Part model, mm, in its own coordinate system. Coordinates: 2 decimals unless noted, no trailing zeros. Order: outer loops, then holes, each group sorted by start corner. A loop starts at its lowest first (then second) coordinate and runs counter-clockwise, first axis right, second up.
1) Pin check, flat tips, straight feed: pin 1 Ø1 at (y, z) = (0, 2.5) entering from -X; pin 2 Ø2.5 at (x, z) = (0, 0) entering from -Y. Stop position of each tip, or through.
2) Cut at A-A (x = 0). List the corners of the cut face in (y, z), and give its area (3 significant figures).
3) Mould opens along X. For faces 1 (the flat face through (2.5, 0, 0.2)), 2 (the cylindrical face through (-11.99, -0.99, 0.53)), 3 (the cylindrical face through (2.003, -0.986, 0.631)) say: +X half, -X half, draft (parallel to the pull), parting line (faces both ways), or undercut.
4) Cut at C-C (y = -0.6). List the corners of the cut face in (x, z).
5) Cut at D-D (x = 10.25). List the corners of the cut face in (y, z), and give its area (3 significant figures).
6) Wall check: L1, parallel to Z at x = 0, y = -1.2; L2, parallel to Z at x = 4.5, y = -0.1; L3, parallel to Z at x = -10.75, y = -1.2. Give the ranges that are in metal, low to high.
7) Cut at B-B (z = 0). List the corners of the cut face in (x, y).
```python
from build123d import *

# Parameters (mm, degrees)
CYLINDER011007_R     = 2.1
CYLINDER011007_DEPTH = 20
CYLINDER011008_R     = 12
CYLINDER011008_DEPTH = 2


with BuildPart() as belt_attach_insert_hole:
    # Cylinder011007 → Cylinder011007 (new body)
    with BuildSketch(Plane.XZ):
        Circle(CYLINDER011007_R)
    extrude(amount=CYLINDER011007_DEPTH)


with BuildPart() as belt_attach_washer_cut:
    # Cylinder011008 → Cylinder011008 (new body)
    with BuildSketch(Plane.XZ):
        Circle(CYLINDER011008_R)
    extrude(amount=CYLINDER011008_DEPTH)

    # Cut023015009008: cut belt attach insert hole
    add(belt_attach_insert_hole.part, mode=Mode.SUBTRACT)


solid = belt_attach_washer_cut.part
```
Geometry check:
1. pin 1: stops at x = -11.83
1. pin 2: passes through
2. outline: (-2, -12) - (0, -12) - (0, -2.1) - (-2, -2.1) - close; (-2, 2.1) - (0, 2.1) - (0, 12) - (-2, 12) - close
2. area: 39.6 mm2
3. face 1: draft
3. face 2: parting line
3. face 3: undercut
4. outline: circle Ø24 at (0, 0); hole circle Ø4.2 at (0, 0)
5. outline: (-2, -6.24) - (0, -6.24) - (0, 6.24) - (-2, 6.24) - close
5. area: 25.0 mm2
6. L1: z = -12 to -2.1, 2.1 to 12
6. L2: z = -11.12 to 11.12
6. L3: z = -5.33 to 5.33
7. outline: (-12, -2) - (-2.1, -2) - (-2.1, 0) - (-12, 0) - close; (2.1, -2) - (12, -2) - (12, 0) - (2.1, 0) - close
